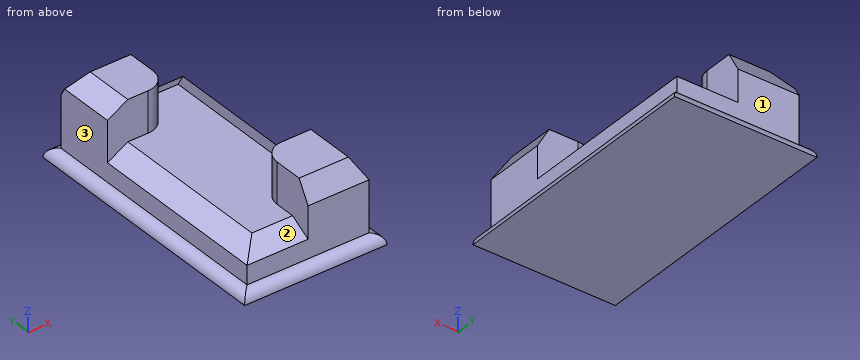
```python
from build123d import *

# Parameters (mm, degrees)
F1_DEPTH    = 50.8
F2_DEPTH    = 25.4
F0_W        = 88.9
F0_H        = 165.1
F3_DEPTH    = 6.35
F4_SIZE2    = 7.3323484187
F4_SIZE     = 12.7
F5_C1_SIZE2 = 7.3323484187
F5_C1_SIZE  = 12.7
F5_C2_SIZE2 = 7.3323484187
F5_C2_SIZE  = 12.7
F5_C3_SIZE2 = 12.7
F5_C3_SIZE  = 7.3323484187
F5_C4_SIZE2 = 7.3323484187
F5_C4_SIZE  = 12.7
F6_R        = 6.34999


# Not quite as in the source:
# - a fillet or chamfer is up to 0.001 mm smaller than in the source, because OpenCascade refuses the exact size


with BuildPart() as f1:
    # F0 (on Top) → F1 (new body)
    with BuildSketch(Plane.XY):
        with BuildLine():
            Line((-19.9555572391, -85.2174787462), (-19.9555572391, -47.1174787462))
            Line((-19.9555572391, -47.1174787462), (-45.3555572391, -47.1174787462))
            ThreePointArc((-45.3555572391, -47.1174787462), (-54.3358133601, -50.8372226251), (-58.0555572391, -59.8174787462))
            Line((-58.0555572391, -59.8174787462), (-58.0555572391, -85.2174787462))
            Line((-58.0555572391, -85.2174787462), (-19.9555572391, -85.2174787462))
        make_face()
    extrude(amount=F1_DEPTH)



with BuildPart() as f1b:
    # F0 (on Top) → F1, piece 2 (new body)
    with BuildSketch(Plane.XY):
        with BuildLine():
            Line((-58.0555572391, 67.1825212538), (-96.1555572391, 67.1825212538))
            Line((-96.1555572391, 67.1825212538), (-96.1555572391, 29.0825212538))
            Line((-96.1555572391, 29.0825212538), (-70.7555572391, 29.0825212538))
            ThreePointArc((-70.7555572391, 29.0825212538), (-61.775301118, 32.8022651328), (-58.0555572391, 41.7825212538))
            Line((-58.0555572391, 41.7825212538), (-58.0555572391, 67.1825212538))
        make_face()
    extrude(amount=F1_DEPTH)


with BuildPart() as f1_1:
    add(f1.part)

    add(f1b.part)  # F2 merges F1b
    # F0 (on Top) → F2 (join)
    with BuildSketch(Plane.XY):
        with BuildLine():
            Line((-19.9555572391, 67.1825212538), (-58.0555572391, 67.1825212538))
            Line((-58.0555572391, 67.1825212538), (-58.0555572391, 41.7825212538))
            ThreePointArc((-58.0555572391, 41.7825212538), (-61.775301118, 32.8022651328), (-70.7555572391, 29.0825212538))
            Line((-70.7555572391, 29.0825212538), (-96.1555572391, 29.0825212538))
            Line((-96.1555572391, 29.0825212538), (-96.1555572391, -85.2174787462))
            Line((-96.1555572391, -85.2174787462), (-58.0555572391, -85.2174787462))
            Line((-58.0555572391, -85.2174787462), (-58.0555572391, -59.8174787462))
            ThreePointArc((-58.0555572391, -59.8174787462), (-54.3358133601, -50.8372226251), (-45.3555572391, -47.1174787462))
            Line((-45.3555572391, -47.1174787462), (-19.9555572391, -47.1174787462))
            Line((-19.9555572391, -47.1174787462), (-19.9555572391, 67.1825212538))
        make_face()
    extrude(amount=F2_DEPTH)

    # F0 (on Top) → F3 (join)
    with BuildSketch(Plane.XY):
        with Locations((-58.0555572391, -9.0174787462)):
            Rectangle(F0_W, F0_H)
        Polygon((-96.1555572391, 29.0825212538), (-96.1555572391, 67.1825212538), (-58.0555572391, 67.1825212538), (-19.9555572391, 67.1825212538), (-19.9555572391, -47.1174787462), (-19.9555572391, -85.2174787462), (-58.0555572391, -85.2174787462), (-96.1555572391, -85.2174787462), align=None, mode=Mode.SUBTRACT)
    extrude(amount=F3_DEPTH)

    # F4
    f4_edges = [f1_1.edges().sort_by_distance(p)[0] for p in [
        (-96.155557, -28.067479, 25.4),
        (-77.105557, -85.217479, 25.4),
        (-19.955557, 10.032521, 25.4),
        (-39.005557, 67.182521, 25.4),
    ]]
    f4_side = f1_1.faces().sort_by_distance((-58.055557, -9.017479, 25.4))[0]
    chamfer(f4_edges, length=F4_SIZE, length2=F4_SIZE2, reference=f4_side)

    # F5: chamfer of 12.7 x 7.3323484187 on 4 edges, made by hand

    # F5_c1
    f5_c1_edges = [f1_1.edges().sort_by_distance(p)[0] for p in [
        (-77.1055572391, 67.1825212538, 50.8),
    ]]
    f5_c1_side = f1_1.faces().sort_by_distance((-77.1055572391, 67.1825212538, 50.6533530316))[0]
    chamfer(f5_c1_edges, length=F5_C1_SIZE, length2=F5_C1_SIZE2, reference=f5_c1_side)

    # F5_c2
    f5_c2_edges = [f1_1.edges().sort_by_distance(p)[0] for p in [
        (-19.9555572391, -66.1674787462, 50.8),
    ]]
    f5_c2_side = f1_1.faces().sort_by_distance((-19.9555572391, -66.1674787462, 50.6533530316))[0]
    chamfer(f5_c2_edges, length=F5_C2_SIZE, length2=F5_C2_SIZE2, reference=f5_c2_side)

    # F5_c3
    f5_c3_edges = [f1_1.edges().sort_by_distance(p)[0] for p in [
        (-96.1555572391, 44.4663470445, 50.8),
    ]]
    f5_c3_side = f1_1.faces().sort_by_distance((-96.1555572391, 44.4663470445, 50.6533530316))[0]
    chamfer(f5_c3_edges, length=F5_C3_SIZE, length2=F5_C3_SIZE2, reference=f5_c3_side)

    # F5_c4
    f5_c4_edges = [f1_1.edges().sort_by_distance(p)[0] for p in [
        (-42.6717314484, -85.2174787462, 50.8),
    ]]
    f5_c4_side = f1_1.faces().sort_by_distance((-42.6717314484, -85.2174787462, 50.6533530316))[0]
    chamfer(f5_c4_edges, length=F5_C4_SIZE, length2=F5_C4_SIZE2, reference=f5_c4_side)

    # F6 (radius 6.35 in the source; OpenCascade refuses exactly that, so slightly less here)
    f6_edges = [f1_1.edges().sort_by_distance(p)[0] for p in [
        (-58.055557, -91.567479, 6.35),
        (-13.605557, -9.017479, 6.35),
        (-102.505557, -9.017479, 6.35),
        (-58.055557, 73.532521, 6.35),
    ]]
    fillet(f6_edges, radius=F6_R)


solid = f1_1.part
```
Here's how the part is built. I have some questions about the finished solid (model axes, mm). Face numbers are marked on the shaded views. A direction names the side the tool comes from. Coordinates: 2 decimals unless noted, no trailing zeros. Write each loop counter-clockwise with the first axis right and the second up, starting at its lowest first coordinate (ties: lowest second). Pieces come first, ordered by that corner, then holes. Notation, with made-up numbers: (35.5, 82.25) -> (79.5, 82.25) arc R21 ccw to (79.5, 115.25) -> close; hole circle Ø3 at (77, 9.5). An arc over 180 degrees is marked (long way). Use a Markdown table: item, result. Add a question column.
(1) If we section it at D-D, the plane z = 10: Write out the boundary of the cut face in (x, y), and give its area (3 significant figures).
(2) I'm going to push flat-ended pins straight in: P1, Ø12, axis at y = 4, z = 19.5, coming from the -X side; P2, Ø4, axis at x = -29, z = 13, coming from the +Y side; P3, Ø2, axis at y = 38, z = 16, coming from the +X side. Where does each tip first touch, or does it pass through?
(3) If we section it at A-A, the plane z = 32.5: Write out the boundary of the cut face in (x, y).
(4) For the marked faces 1, 2 and 3, which set-ups out of +Z, -Z, +X, -X, +Y, -Y let a thin tool reach every point of the face, with its end or its side?
(5) Please list where these lines run through material, in increasing order: line 1 (X direction, y = -60.5, z = 29.5); line 2 (Y direction, x = -70, z = 15.5); line 3 (Z direction, x = -44, y = -1.5).
Outcome:
| question | item | result |
|---|---|---|
| 1 | outline | (-96.16, -85.22) -> (-19.96, -85.22) -> (-19.96, 67.18) -> (-96.16, 67.18) -> close |
| 1 | area | 11,600 mm^2 |
| 2 | P1 | stops at x = -96.16 |
| 2 | P2 | stops at y = 67.18 |
| 2 | P3 | stops at x = -19.96 |
| 3 | outline | (-96.16, 29.08) -> (-70.76, 29.08) arc R12.7 ccw to (-58.06, 41.78) -> (-58.06, 67.18) -> (-96.16, 67.18) -> close; (-58.06, -85.22) -> (-19.96, -85.22) -> (-19.96, -47.12) -> (-45.36, -47.12) arc R12.7 ccw to (-58.06, -59.82) -> close |
| 4 | face 1 | +Z, +X, -X, +Y |
| 4 | face 2 | +Z, -X, -Y |
| 4 | face 3 | +Z, -X, +Y, -Y |
| 5 | line 1 | x = -58.06 to -19.96 |
| 5 | line 2 | y = -85.22 to 67.18 |
| 5 | line 3 | z = 0 to 25.4 |
